Geometry check sheet. Reference: the model listing, model coordinates, mm. Face numbers are marked on the shaded views. A direction names the side the tool comes from. Coordinates: 2 decimals unless noted, no trailing zeros. Write each loop counter-clockwise with the first axis right and the second up, starting at its lowest first coordinate (ties: lowest second). Pieces come first, ordered by that corner, then holes. Notation, with made-up numbers: (46.25, -35) -> (69.25, -35) arc R18 ccw to (69.25, -26) -> close; hole circle Ø1 at (72, 64). An arc over 180 degrees is marked (long way). Put each result on its own line as item: value. Start each with the question number.
from build123d import *

# Parameters (mm, degrees)
F1_DEPTH = 63.5
F0_W     = 25.4
F0_H     = 19.05
F2_DEPTH = 25.4
F3_DEPTH = 7.9375
F4_DEPTH = 25.4
F6_R     = 6.35


with BuildPart() as f1:
    # F0 (on Front) → F1 (new body, symmetric)
    with BuildSketch(Plane.XZ):
        Polygon((-41.275, 9.525), (-41.275, -9.525), (41.275, -9.525), (41.275, 9.525), (22.225, 9.525), align=None)
    extrude(amount=F1_DEPTH, both=True)

    # F0 (on Front) → F2 (join, symmetric)
    with BuildSketch(Plane.XZ):
        with BuildLine():
            Line((22.225, 9.525), (41.275, 9.525))
            Line((41.275, 9.525), (41.275, 27.0002))
            ThreePointArc((41.275, 27.0002), (45.9246798487, 38.2255201513), (57.15, 42.8752))
            Line((57.15, 42.8752), (60.325, 42.8752))
            Line((60.325, 42.8752), (60.325, 61.9252))
            Line((60.325, 61.9252), (57.15, 61.9252))
            add(Edge.make_bspline(
                [(55.8177831664, 61.8997819933), (56.2614415323, 61.9087982491), (56.7055224041, 61.9172649875), (57.15, 61.9252)],
                knots=[110.5462795592, 110.5462795592, 110.5462795592, 110.5462795592, 111.5045361635, 111.5045361635, 111.5045361635, 111.5045361635], degree=3))
            ThreePointArc((55.8177831664, 61.8997819933), (31.9876938864, 51.2203151121), (22.225, 27.0002))
            Line((22.225, 27.0002), (22.225, 9.525))
        make_face()
        with Locations((73.025, 52.4002)):
            Rectangle(F0_W, F0_H)
    extrude(amount=F2_DEPTH, both=True)

    # F0 (on Front) → F3 (join, symmetric)
    with BuildSketch(Plane.XZ):
        with BuildLine():
            add(Edge.make_bspline(
                [(-41.275, 9.525), (-40.9218768846, 52.5063416026), (4.6365217787, 60.8596498155), (55.8177831664, 61.8997819933)],
                knots=[0, 0, 0, 0, 110.5462795592, 110.5462795592, 110.5462795592, 110.5462795592], degree=3))
            Line((-41.275, 9.525), (22.225, 9.525))
            Line((22.225, 9.525), (22.225, 27.0002))
            ThreePointArc((22.225, 27.0002), (31.9876938864, 51.2203151121), (55.8177831664, 61.8997819933))
        make_face()
    extrude(amount=F3_DEPTH, both=True)

    # F0 (on Front) → F4 (join, symmetric)
    with BuildSketch(Plane.XZ):
        with Locations((73.025, 52.4002)):
            Rectangle(F0_W, F0_H)
    extrude(amount=F4_DEPTH, both=True)

    # F0 (on Front) → F5 (revolve)
    with BuildSketch(Plane.XZ):
        Polygon((85.725, 66.675), (85.725, 61.9252), (85.725, 42.8752), (85.725, 38.1), (111.125, 38.1), (111.125, 66.675), align=None)
    revolve(axis=Axis((85.725, 0, 52.3875), (0, 0, 1)))

    # F6
    f6_edges = [f1.edges().sort_by_distance(p)[0] for p in [
        (41.275, -63.5, 0),
        (-41.275, 63.5, 0),
        (-41.275, -63.5, 0),
        (41.275, 63.5, 0),
    ]]
    fillet(f6_edges, radius=F6_R)


solid = f1.part
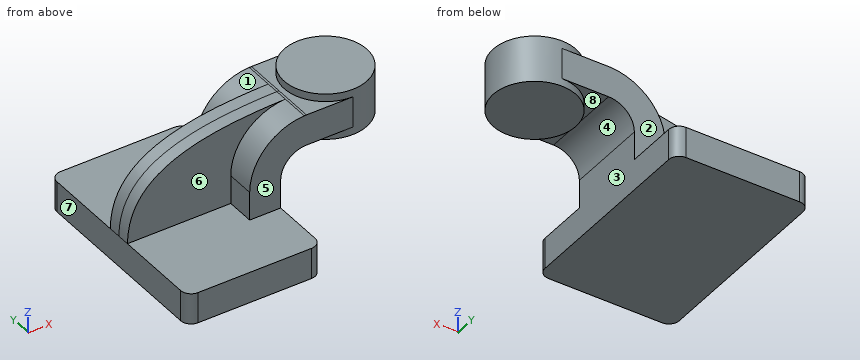
Item 1: Section check C-C, the plane x = 90. Enter the section's corners in (y, z) (3 decimals), and give its area (3 significant figures).
Item 2: Go/stop test with flat-tipped pins: P1, Ø10, axis at y = -19, z = 25, coming from the -X side (3 decimals); P2, Ø10, axis at y = 12, z = 30, coming from the +X side; P3, Ø4, axis at x = 13, z = 58, coming from the -Y side. Record where each tip stops, or that it passes through.
Item 3: Section check A-A, the plane z = 7. Enter the section's corners in (x, y) (3 decimals), and give its area (3 significant figures).
Item 4: Section check B-B, the plane x = 74. Enter the section's corners in (y, z) (3 decimals), and give its area (3 significant figures).
Item 5: Scan lines: line 1 along X through (y, z) = (44, -6) (3 decimals); line 2 along X through (y, z) = (-8, 25) (3 decimals); line 3 along Y through (x, z) = (24, 57). Record each from-to range of solid material in increasing order. Write a range as [from, to].
Item 6: Access from +Z, -Z, +X, -X, +Y, -Y to the whole of each face (thin tool, end or side, straight path). Record for the marked faces 1, 2, 3, 4 and 5.
Item 7: Mould release check, pull along X, two halves, no side actions. Record for the marked faces 6, 7 and 8: released by +X, released by -X, zero draft, split by the parting line, or undercut.
From the geometry:
1. outline: (-25.038, 38.1) -> (25.038, 38.1) -> (25.038, 66.675) -> (-25.038, 66.675) -> close
1. area: 1,430 mm²
2. P1: x = 22.225
2. P2: x = 43.44
2. P3: y = -7.94
3. outline: (-41.275, -57.15) arc R6.35 ccw to (-34.925, -63.5) -> (34.925, -63.5) arc R6.35 ccw to (41.275, -57.15) -> (41.275, 57.15) arc R6.35 ccw to (34.925, 63.5) -> (-34.925, 63.5) arc R6.35 ccw to (-41.275, 57.15) -> close
3. area: 10,400 mm²
4. outline: (-25.4, 42.875) -> (-22.532, 42.875) -> (-22.532, 38.1) -> (22.532, 38.1) -> (22.532, 42.875) -> (25.4, 42.875) -> (25.4, 61.925) -> (22.532, 61.925) -> (22.532, 66.675) -> (-22.532, 66.675) -> (-22.532, 61.925) -> (-25.4, 61.925) -> close
4. area: 1,400 mm²
5. line 1: [-41.275, 41.275]
5. line 2: [22.225, 41.275]
5. line 3: [-7.94, 7.94]
6. face 1: +Z, -X, +Y
6. face 2: +Z, +X, -X, +Y
6. face 3: -Z, +X, +Y, -Y
6. face 4: -Z, +Y, -Y
6. face 5: +Z, +X, -X, -Y
7. face 6: zero draft
7. face 7: released by -X
7. face 8: undercut
